Could you check a few things on this model? Use its own coordinates, in mm. A direction names the side the tool comes from. Give positions to 0.01 mm unless a question says otherwise; leave off trailing zeros. Order: outer loops, then holes, each group sorted by start corner. A loop starts at its lowest first (then second) coordinate and runs counter-clockwise, first axis right, second up. Notation, with made-up numbers: M -29,55.25 L 1,55.25 A27 cw 1,80.25 Z; hole C 16,40 d10. An arc over 180 degrees is marked long. Use a Markdown table: item, result. Add a question column.
Item 1: I'm going to push flat-ended pins straight in: pin 1 Ø10 at (x, z) = (2.5, 40) entering from -Y; pin 2 Ø2.5 at (x, y) = (27, -19) entering from +Z; pin 3 Ø5 at (x, y) = (4.5, 30) entering from -Z; pin 4 Ø22.5 at (y, z) = (-34.5, 33) entering from -X. Where does each tip first touch, or does it pass through?
Item 2: If I drill on L1, parallel to Z at x = -15.5, y = -45.5; L2, parallel to Y at x = -4.5, z = 36; L3, parallel to Z at x = 9.5, y = -21, over which ranges is the centre line in solid material (lowest first)? Write a range as from..to.
Item 3: Suppose I cut it at A-A on x = 21.5. Write out the boundary of the cut face in (y, z).
Item 4: If we mould it in two halves opening along X, with no side actions, what happens to faces 1 (the face through (16, -22.251, 30)), 2 (the face through (38.061, 6, 31)), 3 (the face through (14.061, -42, 8))? For each: released by +X, released by -X, zero draft, split by the parting line, or undercut.
Item 5: Suppose I cut it at B-B on y = 21. Write out the boundary of the cut face in (x, z), plus the area to 3 significant figures.
Item 6: Suppose I cut it at C-C on y = -19.5. Write out the boundary of the cut face in (x, z).
Item 7: For faces 4 (the face through (22, 31, 80)), 5 (the face through (22, 14, 44)), 6 (the face through (6.061, -3, 27)), which set-ups out of +Z, -Z, +X, -X, +Y, -Y let a thin tool reach every point of the face, with its end or its side?
Item 8: Suppose I cut it at D-D on x = 11. Write out the boundary of the cut face in (y, z), plus the area to 3 significant figures.
from build123d import *

# Parameters (mm, degrees)
F0_W      = 64
F0_H      = 96
F1_DEPTH  = 16
F3_DEPTH  = 25
F4_W      = 12
F4_H      = 30
F5_DEPTH  = 28
F7_DEPTH  = 25
F8_W      = 32
F8_H      = 40
F9_DEPTH  = 28
F10_R     = 12
F11_DEPTH = 52
F13_DEPTH = 64
F15_DEPTH = 30


with BuildPart() as f1:
    # F0 (on Top) → F1 (new body)
    with BuildSketch(Plane.XY):
        with Locations((6.061017856, -4.2511862218)):
            Rectangle(F0_W, F0_H)
    extrude(amount=F1_DEPTH)

    # F2 (on face) → F3 (cut)
    with BuildSketch(Plane.XY.offset(16)):
        with BuildLine():
            Line((-1.938982144, -32.2511862218), (-1.938982144, -52.2511862218))
            Line((-1.938982144, -52.2511862218), (14.061017856, -52.2511862218))
            Line((14.061017856, -52.2511862218), (14.061017856, -32.2511862218))
            ThreePointArc((14.061017856, -32.2511862218), (6.061017856, -40.2511862218), (-1.938982144, -32.2511862218))
        make_face()
        with BuildLine():
            ThreePointArc((14.061017856, -32.2511862218), (6.061017856, -24.2511862218), (-1.938982144, -32.2511862218))
            Line((-1.938982144, -32.2511862218), (14.061017856, -32.2511862218))
        make_face()
        with BuildLine():
            Line((14.061017856, -32.2511862218), (-1.938982144, -32.2511862218))
            ThreePointArc((-1.938982144, -32.2511862218), (6.061017856, -40.2511862218), (14.061017856, -32.2511862218))
        make_face()
    extrude(amount=-F3_DEPTH, mode=Mode.SUBTRACT)

    # F4 (on face) → F5 (join)
    with BuildSketch(Plane.XY.offset(16)):
        with Locations((32.061017856, -37.2511862218)):
            Rectangle(F4_W, F4_H)
    extrude(amount=F5_DEPTH)

    # F6 (on face) → F7 (cut)
    with BuildSketch(Plane(origin=(26.061017856, 0, 0), x_dir=(0, -1, 0), z_dir=(-1, 0, 0))):
        Polygon((52.2511862218, 44), (22.2511862218, 44), (52.2511862218, 16), align=None)
    extrude(amount=-F7_DEPTH, mode=Mode.SUBTRACT)

    # F8 (on face) → F9 (join)
    with BuildSketch(Plane.XY.offset(16)):
        with Locations((22.061017856, -2.2511862218)):
            Rectangle(F8_W, F8_H)
    extrude(amount=F9_DEPTH)

    # F10 (on face) → F11 (cut)
    with BuildSketch(Plane(origin=(6.061017856, 0, 0), x_dir=(0, -1, 0), z_dir=(-1, 0, 0))):
        with Locations((2.2511862218, 44)):
            Circle(F10_R)
    extrude(amount=-F11_DEPTH, mode=Mode.SUBTRACT)

    # F12 (on face) → F13 (join)
    with BuildSketch(Plane.XY.offset(16)):
        Polygon((-25.938982144, 17.7488137782), (6.061017856, 17.7488137782), (38.061017856, 17.7488137782), (38.061017856, 43.7488137782), (-25.938982144, 43.7488137782), align=None)
    extrude(amount=F13_DEPTH)

    # F14 (on face) → F15 (cut)
    with BuildSketch(Plane.XZ.offset(-17.7488137782)):
        Polygon((-25.938982144, 50), (6.061017856, 80), (-25.938982144, 80), align=None)
    extrude(amount=-F15_DEPTH, mode=Mode.SUBTRACT)


solid = f1.part
Findings below:
| question | item | result |
|---|---|---|
| 1 | pin 1 | stops at y = -22.25 |
| 1 | pin 2 | stops at z = 44 |
| 1 | pin 3 | stops at z = 0 |
| 1 | pin 4 | stops at x = 26.06 |
| 2 | L1 | z = 0..16 |
| 2 | L2 | y = 17.75..43.75 |
| 2 | L3 | z = 0..44 |
| 3 | outline | M -52.25,0 L 43.75,0 L 43.75,80 L 17.75,80 L 17.75,44 L 9.75,44 A12 cw -14.25,44 L -22.25,44 L -22.25,16 L -52.25,16 Z |
| 4 | face 1 | zero draft |
| 4 | face 2 | released by +X |
| 4 | face 3 | undercut |
| 5 | outline | M -25.94,0 L 38.06,0 L 38.06,80 L 6.06,80 L -25.94,50 Z |
| 5 | area | 4,640 mm^2 |
| 6 | outline | M -25.94,0 L 38.06,0 L 38.06,44 L 6.06,44 L 6.06,16 L -25.94,16 Z |
| 7 | face 4 | +Z, +X, -X, +Y, -Y |
| 7 | face 5 | +Z, +X, -X, -Y |
| 7 | face 6 | +Z, -X, -Y |
| 8 | outline | M -25.96,0 L 43.75,0 L 43.75,80 L 17.75,80 L 17.75,44 L 9.75,44 A12 cw -14.25,44 L -22.25,44 L -22.25,16 L -25.96,16 Z |
| 8 | area | 3,670 mm^2 |
